For this review, take the finished solid that the model builds, in its own axes (mm). A direction names the side the tool comes from. Coordinates: 2 decimals unless noted, no trailing zeros. Order: outer loops, then holes, each group sorted by start corner. A loop starts at its lowest first (then second) coordinate and runs counter-clockwise, first axis right, second up.
from build123d import *

# Parameters (mm, degrees)
BRIDA_BASE1_DEPTH      = 16
CROQUIS6_R             = 1.5
CROQUIS6_W             = 9.788625446
CROQUIS6_H             = 16
CORTAR_EXTRUIR8_DEPTH  = 0.5
CROQUIS10_R            = 1.5
CORTAR_EXTRUIR10_DEPTH = 0.5
CORTAR_EXTRUIR11_DEPTH = 0.5


# Sheet-metal steps are written as plain solids
with BuildPart() as part:
    # Croquis1 → Brida base1 (new body)
    with BuildSketch(Plane(origin=(0, 0, 0), x_dir=(1, 0, 0), z_dir=(0, 1, 0))):
        with BuildLine():
            Line((-58.939086294, 3.693519459), (-58.939086294, -15.306480541))
            ThreePointArc((-58.939086294, -15.306480541), (-58.646193076, -16.013587323), (-57.939086294, -16.306480541))
            Line((-57.939086294, -16.306480541), (2.060913706, -16.306480541))
            ThreePointArc((2.060913706, -16.306480541), (2.768020487, -16.013587323), (3.060913706, -15.306480541))
            Line((3.060913706, -15.306480541), (3.060913706, 3.693519459))
            Line((3.060913706, 3.693519459), (2.560913706, 3.693519459))
            Line((2.560913706, 3.693519459), (2.560913706, -15.306480541))
            ThreePointArc((2.560913706, -15.306480541), (2.414467096, -15.660033932), (2.060913706, -15.806480541))
            Line((2.060913706, -15.806480541), (-57.939086294, -15.806480541))
            ThreePointArc((-57.939086294, -15.806480541), (-58.292639685, -15.660033932), (-58.439086294, -15.306480541))
            Line((-58.439086294, -15.306480541), (-58.439086294, 3.693519459))
            Line((-58.439086294, 3.693519459), (-58.939086294, 3.693519459))
        make_face()
    extrude(amount=BRIDA_BASE1_DEPTH)

    # Croquis6 → Cortar-Extruir8 (cut)
    with BuildSketch(Plane(origin=(3.060913706, 0, 0), x_dir=(0, 0, -1), z_dir=(1, 0, 0))):
        with Locations((-10.095105987, 8.25)):
            Circle(CROQUIS6_R)
        with Locations((-1.200793264, 8)):
            Rectangle(CROQUIS6_W, CROQUIS6_H)
    extrude(amount=-CORTAR_EXTRUIR8_DEPTH, mode=Mode.SUBTRACT)

    # Croquis10 → Cortar-Extruir10 (cut)
    with BuildSketch(Plane.ZY.offset(58.939086294)):
        with BuildLine():
            Line((6.112352523, 11.75), (6.095105987, 16))
            Line((6.095105987, 16), (-3.693519459, 16))
            Line((-3.693519459, 16), (-3.693519459, 0))
            Line((-3.693519459, 0), (6.095105987, 0))
            Line((6.095105987, 0), (9.612352523, 0))
            Line((9.612352523, 0), (9.612352523, 8.25))
            ThreePointArc((9.612352523, 8.25), (8.587226257, 10.724873734), (6.112352523, 11.75))
        make_face()
        with Locations((11.572352523, 8.25)):
            Circle(CROQUIS10_R)
    extrude(amount=-CORTAR_EXTRUIR10_DEPTH, mode=Mode.SUBTRACT)

    # Croquis11 → Cortar-Extruir11 (cut)
    with BuildSketch(Plane.XY.offset(16.306480541)):
        with BuildLine():
            Line((-9.939086294, 12), (-9.939086294, 0))
            Line((-9.939086294, 0), (-4.939086294, 0))
            Line((-4.939086294, 0), (-4.939086294, 12))
            ThreePointArc((-4.939086294, 12), (-7.439086294, 14.5), (-9.939086294, 12))
        make_face()
    extrude(amount=-CORTAR_EXTRUIR11_DEPTH, mode=Mode.SUBTRACT)


solid = part.part
1. The part is to be moulded in two halves that separate along Z. For faces 1 (the face through (-28, 8, 16.306)), 2 (the face through (-58.69, 10.7, 8.61)), 3 (the face through (2.81, 7.34, 11.29)), 4 (the face through (3.061, 8, 12)), say which applies: +Z half, -Z half, draft (parallel to the pull), parting line (faces both ways), or undercut.
Answer below:
face 1: +Z half
face 2: -Z half
face 3: undercut
face 4: draft
2. Take a section at C-C, the plane x = -29. Give the boundary of the cut face in (y, z), plus the area to 3 significant figures.
Answer below:
outline: (0, 15.81) - (16, 15.81) - (16, 16.31) - (0, 16.31) - close
area: 8.00 mm2
3. Take a section at A-A, the plane z = 14.25. Give the boundary of the cut face in (x, y), plus the area to 3 significant figures.
Answer below:
outline: (-58.94, 0) - (-58.44, 0) - (-58.44, 16) - (-58.94, 16) - close; (2.56, 0) - (3.06, 0) - (3.06, 16) - (2.56, 16) - close
area: 16.0 mm2
4. Take a section at B-B, the plane y = 3.75. Give the boundary of the cut face in (x, z), plus the area to 3 significant figures.
Answer below:
outline: (-58.94, 9.61) - (-58.44, 9.61) - (-58.44, 15.31) arc R0.5 cw to (-57.94, 15.81) - (-9.94, 15.81) - (-9.94, 16.31) - (-57.94, 16.31) arc R1 ccw to (-58.94, 15.31) - close; (-4.94, 15.81) - (2.06, 15.81) arc R0.5 cw to (2.56, 15.31) - (2.56, 6.1) - (3.06, 6.1) - (3.06, 15.31) arc R1 ccw to (2.06, 16.31) - (-4.94, 16.31) - close
area: 36.1 mm2
5. Machinability: for faces 5 (the face through (-58.939, 10, 11)), 6 (the face through (-58.439, 10, 11)), 7 (the face through (-58.69, 7.68, 12.96)), which of the approach directions +Z, -Z, +X, -X, +Y, -Y give a long, thin tool a straight path to every point of the face, cutting with its end or side? Answer none if there is none.
Answer below:
face 5: +Z, -Z, -X, +Y, -Y
face 6: -Z, +Y, -Y
face 7: -X
6. To check wall thickness, follow L1, parallel to X at y = 2.25, z = 15; L2, parallel to X at y = 4.75, z = 9.5; L3, parallel to Z at x = -19.5, y = 5. State the ranges of each line that lie inside material, in increasing order.
Answer below:
L1: x = -58.94 to -58.44, 2.56 to 3.06
L2: x = 2.56 to 3.06
L3: z = 15.81 to 16.31
7. Clearance check with flat-ended pins moving along their axes: pin 1 Ø1.5 at (x, y) = (-18, 9.5) entering from -Z; pin 2 Ø1.8 at (y, z) = (8.25, 11.57) entering from -X; pin 3 Ø6 at (x, z) = (-50, 10.5) entering from -Y. State where each tip first meets the part, or that it passes through.
Answer below:
pin 1: stops at z = 15.81
pin 2: stops at x = 2.56
pin 3: passes through
